Check sheet for the drawn part. Datum: minimum x, y, z corner. Units: mm. A direction names the side the tool comes from. Round coordinates to 2 decimals unless told otherwise and drop trailing zeros. Write each loop counter-clockwise with the first axis right and the second up, starting at its lowest first coordinate (ties: lowest second). Pieces come first, ordered by that corner, then holes. Notation, with made-up numbers: M 16,88 L 75,88 A25 ccw 75,124 Z; hole C 84.5,-33.75 d8. An arc over 180 degrees is marked long. Put each result on its own line as item: value.
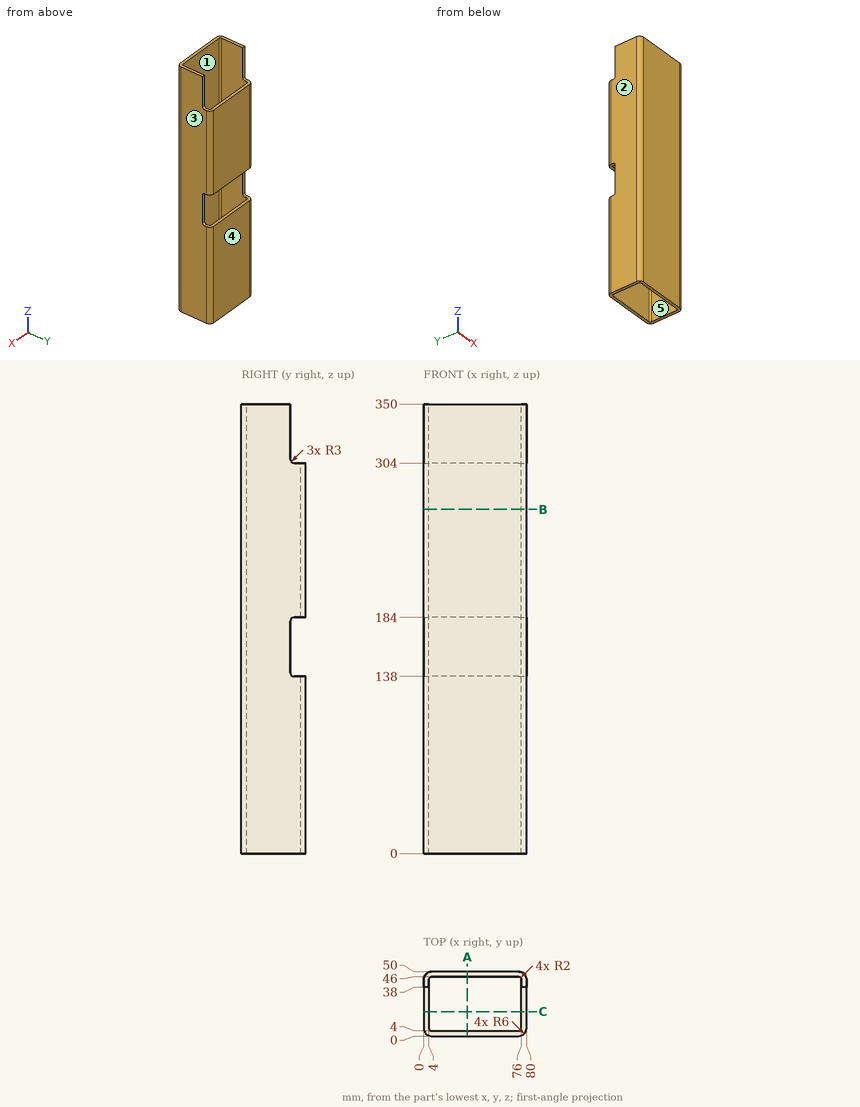
1. Depth check by flat-ended pin: pin 1 Ø12 at (x, y) = (59.5, 5.5) entering from -Z; pin 2 Ø3 at (x, y) = (49, 43.5) entering from -Z; pin 3 Ø4.5 at (x, y) = (36.5, 47.5) entering from +Z; pin 4 Ø1.2 at (x, z) = (77, 163.5) entering from +Y. Enter the tip coordinate at first touch or a pass-through.
Computed values:
pin 1: stops at z = 0
pin 2: passes through
pin 3: stops at z = 304
pin 4: stops at y = 38
2. Cross-section at C-C (y = 19). Enter the section's corners in (x, z), then the cut area to 3 significant figures.
Computed values:
outline: M 0,0 L 4,0 L 4,350 L 0,350 Z; M 76,0 L 80,0 L 80,350 L 76,350 Z
area: 2,800 mm2
3. Access from +Z, -Z, +X, -X, +Y, -Y to the whole of each face (thin tool, end or side, straight path). Record for the marked faces 1 and 2.
Computed values:
face 1: +Z, -Z
face 2: +Z, -Z, -X, +Y, -Y
4. Cross-section at A-A (x = 34). Enter the section's corners in (y, z).
Computed values:
outline: M 0,0 L 4,0 L 4,350 L 0,350 Z; M 46,0 L 50,0 L 50,138 L 46,138 Z; M 46,184 L 50,184 L 50,304 L 46,304 Z
5. Cross-section at B-B (z = 268). Enter the section's corners in (x, y), then the cut area to 3 significant figures.
Computed values:
outline: M 0,6 A6 ccw 6,0 L 74,0 A6 ccw 80,6 L 80,44 A6 ccw 74,50 L 6,50 A6 ccw 0,44 Z; hole M 4,6 A2 ccw 6,4 L 74,4 A2 ccw 76,6 L 76,44 A2 ccw 74,46 L 6,46 A2 ccw 4,44 Z
area: 949 mm2
6. Release check for a two-part mould opening along Y. For the marked faces 3, 4 and 5 record: +Y half, -Y half, draft (parallel to the pull), parting line (faces both ways), or undercut.
Computed values:
face 3: draft
face 4: +Y half
face 5: undercut
7. Scan lines: probe 1 along Y at (x, z) = (21, 198); probe 2 along X at (y, z) = (42.5, 274.5); probe 3 along Y at (x, z) = (37.5, 323). Record each from-to range of solid material in increasing order.
Computed values:
probe 1: y = 0 to 4, 46 to 50
probe 2: x = 0 to 4, 76 to 80
probe 3: y = 0 to 4
